```python
from build123d import *

# Parameters (mm, degrees)
SKETCH1_R           = 2.7
BOSS_EXTRUDE1_DEPTH = 13
FILLET1_R           = 0.8


with BuildPart() as part:
    # Sketch1 → Boss-Extrude1 (new body)
    with BuildSketch(Plane(origin=(0, 0, 0), x_dir=(1, 0, 0), z_dir=(0, 1, 0))):
        with BuildLine():
            Line((51.921017872, 32.018867925), (0, 53))
            ThreePointArc((0, 53), (-4, 49), (0, 45))
            ThreePointArc((0, 45), (42.286167935, 15.39090645), (28.925442436, -34.47199994))
            ThreePointArc((28.925442436, -34.47199994), (28.432415102, -40.107328152), (34.067743313, -40.600355485))
            Line((34.067743313, -40.600355485), (31.496592875, -37.536177713))
            ThreePointArc((31.496592875, -37.536177713), (48.373872913, -7.808227676), (41.707047143, 25.720074234))
            Line((41.707047143, 25.720074234), (51.921017872, 32.018867925))
        make_face()
        with Locations((0, 49)):
            Circle(SKETCH1_R, mode=Mode.SUBTRACT)
    extrude(amount=BOSS_EXTRUDE1_DEPTH)

    # Fillet1
    fillet1_edges = [part.edges().sort_by_distance(p)[0] for p in [
        (51.921017872, 6.5, -32.018867925),
        (41.707047143, 6.5, -25.720074234),
        (31.496592875, 6.5, 37.536177713),
        (34.067743313, 6.5, 40.600355485),
        (0, 6.5, -53),
    ]]
    fillet(fillet1_edges, radius=FILLET1_R)


solid = part.part
```
Geometry: final body of the model. Coordinates: model frame, mm. A direction names the side the tool comes from. Coordinates: 2 decimals unless noted, no trailing zeros. Order: outer loops, then holes, each group sorted by start corner. A loop starts at its lowest first (then second) coordinate and runs counter-clockwise, first axis right, second up. Notation, with made-up numbers: (-37, -16.75) -> (22, -16.75) arc R28 cw to (22, 9.25) -> close; hole circle Ø10 at (-29, 17). An arc over 180 degrees is marked (long way). Use CSV: the item, a comma, the result in double quotes.
1) Line query: line 1 (Z direction, x = 0, y = 9.25); line 2 (X direction, y = 9.5, z = -47); line 3 (X direction, y = 3.25, z = -49). Output: solid intervals per line, ascending.
Findings:
line 1,"z = -52.98 to -51.7, -46.3 to -45"
line 2,"x = -3.46 to -1.81, 1.81 to 14.85"
line 3,"x = -4 to -2.7, 2.7 to 9.9"
2) Pin query (flat end, axial travel): pin 1 Ø1 at (x, y) = (2, 10) entering from -Z; pin 2 Ø6 at (y, z) = (10, 13) entering from -X; pin 3 Ø4 at (x, y) = (34.5, 9) entering from +Z. Return the tip coordinate at first contact, or that it passes through.
Findings:
pin 1,"stops at z = -52.39"
pin 2,"stops at x = 42.06"
pin 3,"stops at z = 41.41"
3) Mould query, pull axis X, two halves, no side actions, for faces 1 (the cylindrical face through (-4, 6, -49)), 2 (the cylindrical face through (1.246, 6.409, -46.605)), 3 (the flat face through (46.421, 6.409, -28.627)). Classes: +X half, -X half, draft (parallel to the pull), parting line (faces both ways), or undercut.
Findings:
face 1,"-X half"
face 2,"undercut"
face 3,"+X half"
4) Section D-D on z = 27.5. Output: boundary loops of the cut face in (x, y), then the cut area to 3 significant figures.
Findings:
outline,"(35.62, 0) -> (40.56, 0) -> (40.56, 13) -> (35.62, 13) -> close"
area,"64.2 mm^2"
5) Section C-C on x = 23.5. Output: boundary loops of the cut face in (y, z).
Findings:
outline,"(0, -43.5) -> (13, -43.5) -> (13, -38.38) -> (0, -38.38) -> close"
6) Section B-B on y = 1. Output: boundary loops of the cut face in (x, z).
Findings:
outline,"(-0.18, -53) arc R0.8 ccw to (0.15, -52.94) -> (50.45, -32.61) arc R0.8 ccw to (50.57, -31.19) -> (42.38, -26.14) arc R0.8 cw to (42.11, -25.05) arc R49 ccw to (32.1, 37.03) arc R0.8 cw to (32.01, 38.14) -> (33.49, 39.91) arc R0.8 ccw to (33.22, 41.15) arc R4 ccw to (28.93, 34.47) arc R45 cw to (0, -45) arc R4 ccw to start; hole circle Ø5.4 at (0, -49)"
7) Section A-A on z = -49. Output: boundary loops of the cut face in (x, y).
Findings:
outline,"(-4, 0) -> (-2.7, 0) -> (-2.7, 13) -> (-4, 13) -> close; (2.7, 0) -> (9.9, 0) -> (9.9, 13) -> (2.7, 13) -> close"
8) Access query for faces 4 (the cylindrical face through (42.017, 6.409, -16.112)), 5 (the flat face through (32.76, 6.41, 39.04)). Directions: +Z, -Z, +X, -X, +Y, -Y. A direction counts if a zero-diameter tool reaches every point of the face in a straight line with its end or side. Return the directions, or none.
Findings:
face 4,"-X, +Y, -Y"
face 5,"+X, +Y, -Y"
